Here's how the part is built. I have some questions about the finished solid (model axes, mm). A direction names the side the tool comes from. Give positions to 0.01 mm unless a question says otherwise; leave off trailing zeros. Loops run counter-clockwise (first coordinate to the right, second up) from the corner with the lowest first, then second, coordinate; pieces in that order, holes last. Notation, with made-up numbers: (-34.5, 52.5) -> (-3.5, 52.5) arc R18 ccw to (-3.5, 84.5) -> close; hole circle Ø2 at (40, -22). An arc over 180 degrees is marked (long way). Answer in a Markdown table with one row per item. Add a question column.
Item 1: Which directions (+Z, -Z, +X, -X, +Y, -Y) give clear straight access to the entire face, cutting with the end or side of a thin tool? Please do faces 4 (the face through (-12.5, -1, -5)), 5 (the face through (12.5, -1, -5)), 6 (the face through (2.1, 4.9, -3.5)).
Item 2: If we section it at C-C (x = -0.5): Write out the boundary of the cut face in (y, z).
Item 3: For P1, Ø11, axis at x = -0.5, y = 7.5, coming from the +Z side; P2, Ø19, axis at x = 36, y = 16, coming from the -Z side; P3, Ø1.5, axis at y = 15, z = -4.5, coming from the -X side, each with a flat end and sliding along its axis, tell me the tip position at first contact or that it passes through.
Item 4: We'd pull the mould along X, two halves only. Please class faces 1 (the face through (-2.302, 1.777, -0.542)), 2 (the face through (-1, 1, 2.5)), 3 (the face through (-50, -1, 0)): released by +X, released by -X, zero draft, split by the parting line, or undercut.
Item 5: If we section it at A-A (z = 0): Write out the boundary of the cut face in (x, y), then the cut area to 3 significant figures.
Item 6: If I drill on line 1 (X direction, y = -35, z = 0.05); line 2 (Y direction, x = -0.5, z = -5.75); line 3 (Y direction, x = -0.5, z = 0.8), over which ranges is the centre line in solid material (lowest first)?
Item 7: If we section it at B-B (y = 35): Write out the boundary of the cut face in (x, z).
Item 8: If we section it at D-D (y = -7.5): Write out the boundary of the cut face in (x, z), then the cut area to 3 significant figures.
Autodesk Inventor part; units mm, degrees
ref_plane "YZ Plane" through (0, 0, 0) normal (1, 0, 0) x (0, 1, 0)
ref_plane "XZ Plane" through (0, 0, 0) normal (0, 1, 0) x (-1, 0, 0)
ref_plane "XY Plane" through (0, 0, 0) normal (0, 0, 1) x (1, 0, 0)
sketch "Sketch4" plane through (0, 0, 0) normal (0, 0, 1) x (1, 0, 0)
  line L0 (-50, 50) -> (50, 50)
  line L1 (50, 50) -> (50, -50)
  line L2 (50, -50) -> (-50, -50)
  line L3 (-50, -50) -> (-50, 50)
  line L4 (-50, 50) -> (50, -50) construction
  line L5 (50, 50) -> (-50, -50) construction
  point P0 (0, 0)
  dimension "d34" = 100
  dimension "d35" = 100
extrude "Extrusion2" add sketch "Sketch4" along normal mid plane 5
sketch "Sketch5" plane through (-50, -50, 2.5) normal (0, -1, 0) x (1, 0, 0)
  line L0 (0, -5) -> (100, -5)
  line L1 (37.5, -5) -> (62.5, -5)
  line L2 (62.5, -5) -> (62.5, -10)
  line L3 (62.5, -10) -> (37.5, -10)
  line L4 (37.5, -10) -> (37.5, -5)
  line L5 (100, -5) -> (0, -5)
  point P0 (50, -2.5)
  point P1 (50, -5)
  point P2 (62.5, -7.5)
  point P3 (37.5, -7.5)
  point P4 (50, -5)
  dimension "d38" = 25
  dimension "d39" = 12.5
  dimension "d40" = 5
extrude "Extrusion3" add sketch "Sketch5" against normal up to surface (100 mm away)
sketch "Sketch6" plane through (0, 0, 2.5) normal (0, 0, 1) x (1, 0, 0)
  circle A0 centre (-0.5, 7.5) radius 2.4585
  line L0 (-12.5, 13.5) -> (12.5, 13.5)
  circle A1 centre (-0.5, -7.5) radius 2.4585
  point P0 (0, 0)
hole "Hole3" at (-0.5, -7.5, 2.5) at (-0.5, 7.5, 2.5) direction (0, 0, -1) diameter 7 depth 10 tip angle 118 counterbore diameter 12 counterbore depth 6
sketch "Sketch7" plane through (0, 0, 2.5) normal (0, 0, 1) x (1, 0, 0)
  line L0 (50, -50) -> (50, 50)
  line L1 (-50, -50) -> (50, -50)
  line L2 (50, 50) -> (-50, 50)
  line L3 (-50, 50) -> (-50, -50)
  point P0 (0, 0)
  point P1 (35, -35)
  point P2 (-35, -35)
  point P3 (-35, 35)
  point P4 (35, 35)
  dimension "d50" = 15
  dimension "d51" = 15
  dimension "d52" = 15
  dimension "d53" = 15
hole "Hole4" at (35, -35, 2.5) at (-35, -35, 2.5) at (-35, 35, 2.5) at (35, 35, 2.5) direction (0, 0, -1) diameter 4.134 depth 14.2 tip angle 118
sketch "Sketch1" plane through (0, 0, 0) normal (0, 1, 0) x (-1, 0, 0)
  line L0 (65, -7.5) -> (-65, -7.5)
  line L1 (-65, -7.5) -> (-65, -7.5)
  line L2 (-65, -7.5) -> (-65, -7.5)
  line L3 (-65, -7.5) -> (-65, 2.5)
  line L4 (-65, 2.5) -> (-35, 2.5)
  line L5 (-35, 2.5) -> (-35, -2.5)
  line L6 (-35, -2.5) -> (65, -2.5)
  line L7 (65, -2.5) -> (65, -7.5)
  point P0 (0, 0)
  dimension "d0" = 130
  dimension "d1" = 130
  dimension "d2" = 30
  dimension "d5" = 5
  dimension "d6" = 5
  dimension "d7" = 10
  dimension "d8" = 65
  dimension "d9" = 7.5
sketch "Sketch3" plane through (65, 40, -7.5) normal (0, 0, -1) x (-1, 0, 0)
  line L0 (0, 0) -> (130, 0)
  line L1 (0, -80) -> (0, 0)
  point P0 (65, -40)
  point P1 (65, -40)
  point P2 (12, -32.5)
  point P3 (12, -47.5)
  dimension "d23" = 15
  dimension "d25" = 32.5
  dimension "d26" = 12
properties part number "HCMUTE-CDT23-BAN_CAN_LOADCELL" material "Stainless Steel"
Recorded:
| question | item | result |
|---|---|---|
| 1 | face 4 | -Z, -X, +Y, -Y |
| 1 | face 5 | -Z, +X, +Y, -Y |
| 1 | face 6 | +Z |
| 2 | outline | (-50, -7.5) -> (-11, -7.5) -> (-11, -3.5) -> (-13.5, -3.5) -> (-13.5, 2.5) -> (-50, 2.5) -> close; (-4, -7.5) -> (4, -7.5) -> (4, -3.5) -> (1.5, -3.5) -> (1.5, 2.5) -> (-1.5, 2.5) -> (-1.5, -3.5) -> (-4, -3.5) -> close; (11, -7.5) -> (50, -7.5) -> (50, 2.5) -> (13.5, 2.5) -> (13.5, -3.5) -> (11, -3.5) -> close |
| 3 | P1 | stops at z = -3.5 |
| 3 | P2 | stops at z = -2.5 |
| 3 | P3 | stops at x = -12.5 |
| 4 | face 1 | undercut |
| 4 | face 2 | zero draft |
| 4 | face 3 | released by -X |
| 5 | outline | (-50, -50) -> (50, -50) -> (50, 50) -> (-50, 50) -> close; hole circle Ø4.13 at (-35, -35); hole circle Ø4.13 at (-35, 35); hole circle Ø12 at (-0.5, -7.5); hole circle Ø12 at (-0.5, 7.5); hole circle Ø4.13 at (35, -35); hole circle Ø4.13 at (35, 35) |
| 5 | area | 9,720 mm^2 |
| 6 | line 1 | x = -50 to -37.07, -32.93 to 32.93, 37.07 to 50 |
| 6 | line 2 | y = -50 to -11, -4 to 4, 11 to 50 |
| 6 | line 3 | y = -50 to -13.5, -1.5 to 1.5, 13.5 to 50 |
| 7 | outline | (-50, -2.5) -> (-37.07, -2.5) -> (-37.07, 2.5) -> (-50, 2.5) -> close; (-32.93, -2.5) -> (-12.5, -2.5) -> (-12.5, -7.5) -> (12.5, -7.5) -> (12.5, -2.5) -> (32.93, -2.5) -> (32.93, 2.5) -> (-32.93, 2.5) -> close; (37.07, -2.5) -> (50, -2.5) -> (50, 2.5) -> (37.07, 2.5) -> close |
| 8 | outline | (-50, -2.5) -> (-12.5, -2.5) -> (-12.5, -7.5) -> (-4, -7.5) -> (-4, -3.5) -> (-6.5, -3.5) -> (-6.5, 2.5) -> (-50, 2.5) -> close; (3, -7.5) -> (12.5, -7.5) -> (12.5, -2.5) -> (50, -2.5) -> (50, 2.5) -> (5.5, 2.5) -> (5.5, -3.5) -> (3, -3.5) -> close |
| 8 | area | 525 mm^2 |
